Here's how the part is built. I have some questions about the finished solid (model axes, mm). A direction names the side the tool comes from. Round coordinates to 2 decimals unless told otherwise and drop trailing zeros. Write each loop counter-clockwise with the first axis right and the second up, starting at its lowest first coordinate (ties: lowest second). Pieces come first, ordered by that corner, then holes. Notation, with made-up numbers: (-35, -32.75) -> (-16, -32.75) arc R8 ccw to (-16, -23.75) -> close; hole circle Ø4 at (46.25, 55.25). An arc over 180 degrees is marked (long way). Put each result on its own line as item: value. Start each with the question number.
1. Suppose I cut it at C-C (y = -6). Please give me the cut outline in (x, z), then the cut area to 3 significant figures.
2. Suppose I cut it at B-B (y = -0.25). Please give me the cut outline in (x, z), then the cut area to 3 significant figures.
3. Which directions (+Z, -Z, +X, -X, +Y, -Y) give clear straight access to the entire face, cutting with the end or side of a thin tool? Please do faces 1 (the face through (5.51, -0.16, 2.13)), 2 (the face through (-4, -5, 7.12)), 3 (the face through (-3.99, -6.91, 8.03)), 4 (the face through (-2, 3.95, 5)), 5 (the face through (6, -3, 5)).
4. For pin 1 (0.5 mm diameter, centred on x = -1, y = 0, fed in from -Z); pin 2 (5 mm diameter, centred on x = -1, z = 3.5, fed in from -Y); pin 3 (0.8 mm diameter, centred on y = -5, z = 2.5, fed in from -X); pin 4 (1.9 mm diameter, centred on y = 1.5, z = 3.5, fed in from +X), each with a flat end and sliding along its axis, tell me the tip position at first contact or that it passes through.
5. I need wall thicknesses on probe 1 along Y at (x, z) = (1, 3); probe 2 along Y at (x, z) = (0.5, 7.5); probe 3 along Z at (x, y) = (3.5, -2.5). Which ranges of each line are inside material? Lowest first, please. Write a range as from..to.
6. We'd pull the mould along Z, two halves only. Please class faces 6 (the face through (-4, -5, 8.12)), 7 (the face through (2, 3.45, 5)), 8 (the face through (-4.5, -5.2, 7.6)): +Z half, -Z half, draft (parallel to the pull), parting line (faces both ways), or undercut.
7. Suppose I cut it at D-D (x = -4). Please give me the cut outline in (y, z), then the cut area to 3 significant figures.
8. Suppose I cut it at A-A (x = -2.75). Please give me the cut outline in (y, z).
```python
from build123d import *

# Parameters (mm, degrees)
SKIZZE3_W                       = 12
SKIZZE3_H                       = 7.9
AUFSATZ_LINEAR_AUSTRAGEN2_DEPTH = 10.16
AUFSATZ_LINEAR_AUSTRAGEN3_DEPTH = 10.16
SCHNITT_LINEAR_AUSTRAGEN1_DEPTH = 9
SKIZZE6_W                       = 1
SKIZZE6_H                       = 1
AUFSATZ_LINEAR_AUSTRAGEN4_DEPTH = 3.45
SKIZZE7_W                       = 1
SKIZZE7_H                       = 1
AUFSATZ_LINEAR_AUSTRAGEN5_DEPTH = 9
FASE1_SIZE                      = 1
FASE1_SIZE2                     = 0.176326981
FASE1_PART_2_SIZE               = 1
FASE1_PART_2_SIZE2              = 0.176326981
FASE1_PART_3_SIZE               = 1
FASE1_PART_3_SIZE2              = 0.176326981
FASE1_PART_4_SIZE               = 1
FASE1_PART_4_SIZE2              = 0.176326981
FASE1_PART_5_SIZE               = 1
FASE1_PART_5_SIZE2              = 0.176326981
FASE1_PART_6_SIZE               = 1
FASE1_PART_6_SIZE2              = 0.176326981
FASE1_PART_7_SIZE               = 1
FASE1_PART_7_SIZE2              = 0.176326981
FASE1_PART_8_SIZE               = 1
FASE1_PART_8_SIZE2              = 0.176326981
FASE14_SIZE                     = 1
FASE14_SIZE2                    = 0.176326981
FASE14_PART_2_SIZE              = 1
FASE14_PART_2_SIZE2             = 0.176326981
FASE14_PART_3_SIZE              = 1
FASE14_PART_3_SIZE2             = 0.176326981
FASE14_PART_4_SIZE              = 1
FASE14_PART_4_SIZE2             = 0.176326981
FASE14_PART_5_SIZE              = 1
FASE14_PART_5_SIZE2             = 0.176326981
FASE14_PART_6_SIZE              = 1
FASE14_PART_6_SIZE2             = 0.176326981
FASE14_PART_7_SIZE              = 1
FASE14_PART_7_SIZE2             = 0.176326981
FASE14_PART_8_SIZE              = 1
FASE14_PART_8_SIZE2             = 0.176326981
FASE15_SIZE                     = 0.1
FASE16_SIZE                     = 0.5


with BuildPart() as part:
    # Skizze3 → Aufsatz-Linear austragen2 (new body)
    with BuildSketch(Plane.XY):
        Rectangle(SKIZZE3_W, SKIZZE3_H)
    extrude(amount=AUFSATZ_LINEAR_AUSTRAGEN2_DEPTH)

    # Skizze4 → Aufsatz-Linear austragen3 (add, through all)
    with BuildSketch(Plane.XY.offset(10.16)):
        Polygon((3, 3.95), (3, 4.45), (4, 4.45), (6, 3.95), align=None)
    extrude(amount=-AUFSATZ_LINEAR_AUSTRAGEN3_DEPTH)

    # Skizze5 → Schnitt-Linear austragen1 (cut)
    with BuildSketch(Plane(origin=(6, 0, 0), x_dir=(0, 0, -1), z_dir=(1, 0, 0))):
        with BuildLine():
            Line((-9.86, 3.45), (-9.86, -1.39))
            ThreePointArc((-9.86, -1.39), (-7.602375704, -2.785098012), (-5.08, -1.96))
            ThreePointArc((-5.08, -1.96), (-2.557624296, -2.785098012), (-0.3, -1.39))
            Line((-0.3, -1.39), (-0.3, 3.45))
            Line((-0.3, 3.45), (-9.86, 3.45))
        make_face()
    extrude(amount=-SCHNITT_LINEAR_AUSTRAGEN1_DEPTH, mode=Mode.SUBTRACT)

    # Skizze6 → Aufsatz-Linear austragen4 (add)
    with BuildSketch(Plane(origin=(0, -3.95, 0), x_dir=(-1, 0, 0), z_dir=(0, -1, 0))):
        with Locations((4, -7.62)):
            Rectangle(SKIZZE6_W, SKIZZE6_H)
        with Locations((4, -2.54)):
            Rectangle(SKIZZE6_W, SKIZZE6_H)
    extrude(amount=AUFSATZ_LINEAR_AUSTRAGEN4_DEPTH)

    # Skizze7 → Aufsatz-Linear austragen5 (add)
    with BuildSketch(Plane(origin=(-3, 0, 0), x_dir=(0, 0, -1), z_dir=(1, 0, 0))):
        with Locations((-7.62, -0.15)):
            Rectangle(SKIZZE7_W, SKIZZE7_H)
        with Locations((-2.54, -0.15)):
            Rectangle(SKIZZE7_W, SKIZZE7_H)
    extrude(amount=AUFSATZ_LINEAR_AUSTRAGEN5_DEPTH)

    # Fase1
    fase1_edges = [part.edges().sort_by_distance(p)[0] for p in [
        (-3.5, -7.4, 7.62),
    ]]
    fase1_side = [part.faces().sort_by_distance(p)[0] for p in [
        (-3.5, -5.675, 7.62),
    ]]
    chamfer(fase1_edges, length=FASE1_SIZE, length2=FASE1_SIZE2, reference=fase1_side[0])

    # Fase1 part 2
    fase1_part_2_edges = [part.edges().sort_by_distance(p)[0] for p in [
        (-4, -7.4, 8.12),
    ]]
    fase1_part_2_side = [part.faces().sort_by_distance(p)[0] for p in [
        (-4, -5.675, 8.12),
    ]]
    chamfer(fase1_part_2_edges, length=FASE1_PART_2_SIZE, length2=FASE1_PART_2_SIZE2, reference=fase1_part_2_side[0])

    # Fase1 part 3
    fase1_part_3_edges = [part.edges().sort_by_distance(p)[0] for p in [
        (-4.5, -7.4, 7.62),
    ]]
    fase1_part_3_side = [part.faces().sort_by_distance(p)[0] for p in [
        (-4.5, -5.675, 7.62),
    ]]
    chamfer(fase1_part_3_edges, length=FASE1_PART_3_SIZE, length2=FASE1_PART_3_SIZE2, reference=fase1_part_3_side[0])

    # Fase1 part 4
    fase1_part_4_edges = [part.edges().sort_by_distance(p)[0] for p in [
        (-4, -7.4, 7.12),
    ]]
    fase1_part_4_side = [part.faces().sort_by_distance(p)[0] for p in [
        (-4, -5.675, 7.12),
    ]]
    chamfer(fase1_part_4_edges, length=FASE1_PART_4_SIZE, length2=FASE1_PART_4_SIZE2, reference=fase1_part_4_side[0])

    # Fase1 part 5
    fase1_part_5_edges = [part.edges().sort_by_distance(p)[0] for p in [
        (-4.5, -7.4, 2.54),
    ]]
    fase1_part_5_side = [part.faces().sort_by_distance(p)[0] for p in [
        (-4.5, -5.675, 2.54),
    ]]
    chamfer(fase1_part_5_edges, length=FASE1_PART_5_SIZE, length2=FASE1_PART_5_SIZE2, reference=fase1_part_5_side[0])

    # Fase1 part 6
    fase1_part_6_edges = [part.edges().sort_by_distance(p)[0] for p in [
        (-4, -7.4, 2.04),
    ]]
    fase1_part_6_side = [part.faces().sort_by_distance(p)[0] for p in [
        (-4, -5.675, 2.04),
    ]]
    chamfer(fase1_part_6_edges, length=FASE1_PART_6_SIZE, length2=FASE1_PART_6_SIZE2, reference=fase1_part_6_side[0])

    # Fase1 part 7
    fase1_part_7_edges = [part.edges().sort_by_distance(p)[0] for p in [
        (-3.5, -7.4, 2.54),
    ]]
    fase1_part_7_side = [part.faces().sort_by_distance(p)[0] for p in [
        (-3.5, -5.675, 2.54),
    ]]
    chamfer(fase1_part_7_edges, length=FASE1_PART_7_SIZE, length2=FASE1_PART_7_SIZE2, reference=fase1_part_7_side[0])

    # Fase1 part 8
    fase1_part_8_edges = [part.edges().sort_by_distance(p)[0] for p in [
        (-4, -7.4, 3.04),
    ]]
    fase1_part_8_side = [part.faces().sort_by_distance(p)[0] for p in [
        (-4, -5.675, 3.04),
    ]]
    chamfer(fase1_part_8_edges, length=FASE1_PART_8_SIZE, length2=FASE1_PART_8_SIZE2, reference=fase1_part_8_side[0])

    # Fase14
    fase14_edges = [part.edges().sort_by_distance(p)[0] for p in [
        (6, -0.65, 7.62),
    ]]
    fase14_side = [part.faces().sort_by_distance(p)[0] for p in [
        (1.5, -0.65, 7.62),
    ]]
    chamfer(fase14_edges, length=FASE14_SIZE, length2=FASE14_SIZE2, reference=fase14_side[0])

    # Fase14 part 2
    fase14_part_2_edges = [part.edges().sort_by_distance(p)[0] for p in [
        (6, -0.15, 8.12),
    ]]
    fase14_part_2_side = [part.faces().sort_by_distance(p)[0] for p in [
        (1.5, -0.15, 8.12),
    ]]
    chamfer(fase14_part_2_edges, length=FASE14_PART_2_SIZE, length2=FASE14_PART_2_SIZE2, reference=fase14_part_2_side[0])

    # Fase14 part 3
    fase14_part_3_edges = [part.edges().sort_by_distance(p)[0] for p in [
        (6, 0.35, 7.62),
    ]]
    fase14_part_3_side = [part.faces().sort_by_distance(p)[0] for p in [
        (1.5, 0.35, 7.62),
    ]]
    chamfer(fase14_part_3_edges, length=FASE14_PART_3_SIZE, length2=FASE14_PART_3_SIZE2, reference=fase14_part_3_side[0])

    # Fase14 part 4
    fase14_part_4_edges = [part.edges().sort_by_distance(p)[0] for p in [
        (6, -0.15, 7.12),
    ]]
    fase14_part_4_side = [part.faces().sort_by_distance(p)[0] for p in [
        (1.5, -0.15, 7.12),
    ]]
    chamfer(fase14_part_4_edges, length=FASE14_PART_4_SIZE, length2=FASE14_PART_4_SIZE2, reference=fase14_part_4_side[0])

    # Fase14 part 5
    fase14_part_5_edges = [part.edges().sort_by_distance(p)[0] for p in [
        (6, -0.15, 3.04),
    ]]
    fase14_part_5_side = [part.faces().sort_by_distance(p)[0] for p in [
        (1.5, -0.15, 3.04),
    ]]
    chamfer(fase14_part_5_edges, length=FASE14_PART_5_SIZE, length2=FASE14_PART_5_SIZE2, reference=fase14_part_5_side[0])

    # Fase14 part 6
    fase14_part_6_edges = [part.edges().sort_by_distance(p)[0] for p in [
        (6, 0.35, 2.54),
    ]]
    fase14_part_6_side = [part.faces().sort_by_distance(p)[0] for p in [
        (1.5, 0.35, 2.54),
    ]]
    chamfer(fase14_part_6_edges, length=FASE14_PART_6_SIZE, length2=FASE14_PART_6_SIZE2, reference=fase14_part_6_side[0])

    # Fase14 part 7
    fase14_part_7_edges = [part.edges().sort_by_distance(p)[0] for p in [
        (6, -0.15, 2.04),
    ]]
    fase14_part_7_side = [part.faces().sort_by_distance(p)[0] for p in [
        (1.5, -0.15, 2.04),
    ]]
    chamfer(fase14_part_7_edges, length=FASE14_PART_7_SIZE, length2=FASE14_PART_7_SIZE2, reference=fase14_part_7_side[0])

    # Fase14 part 8
    fase14_part_8_edges = [part.edges().sort_by_distance(p)[0] for p in [
        (6, -0.65, 2.54),
    ]]
    fase14_part_8_side = [part.faces().sort_by_distance(p)[0] for p in [
        (1.5, -0.65, 2.54),
    ]]
    chamfer(fase14_part_8_edges, length=FASE14_PART_8_SIZE, length2=FASE14_PART_8_SIZE2, reference=fase14_part_8_side[0])

    # Fase15
    fase15_edges = [part.edges().sort_by_distance(p)[0] for p in [
        (6, 3.45, 5.08),
        (6, -2.785098012, 7.602375704),
        (6, -2.785098012, 2.557624296),
    ]]
    chamfer(fase15_edges, length=FASE15_SIZE)

    # Fase16
    fase16_edges = [part.edges().sort_by_distance(p)[0] for p in [
        (6, -3.95, 5.08),
    ]]
    chamfer(fase16_edges, length=FASE16_SIZE)


solid = part.part
```
Verdict:
1. outline: (-4.5, 2.04) -> (-3.5, 2.04) -> (-3.5, 3.04) -> (-4.5, 3.04) -> close; (-4.5, 7.12) -> (-3.5, 7.12) -> (-3.5, 8.12) -> (-4.5, 8.12) -> close
1. area: 2.00 mm^2
2. outline: (-6, 0) -> (6, 0) -> (6, 0.3) -> (-3, 0.3) -> (-3, 2.04) -> (5, 2.04) -> (6, 2.22) -> (6, 2.86) -> (5, 3.04) -> (-3, 3.04) -> (-3, 7.12) -> (5, 7.12) -> (6, 7.3) -> (6, 7.94) -> (5, 8.12) -> (-3, 8.12) -> (-3, 9.86) -> (6, 9.86) -> (6, 10.16) -> (-6, 10.16) -> close
2. area: 53.5 mm^2
3. face 1: +X
3. face 2: +X, -X, -Y
3. face 3: +Z, +X, -X, -Y
3. face 4: +Z, -Z, -X, +Y
3. face 5: +Z, -Z, +X, +Y, -Y
4. pin 1: stops at z = 0
4. pin 2: stops at y = -3.95
4. pin 3: stops at x = -4.5
4. pin 4: stops at x = -3
5. probe 1: y = -3.95..-2.81, -0.65..0.35, 3.45..3.95
5. probe 2: y = -3.95..-2.8, -0.65..0.35, 3.45..3.95
5. probe 3: z = 0..1.57, 4.29..5.87, 8.59..10.16
6. face 6: +Z half
6. face 7: undercut
6. face 8: draft
7. outline: (-7.4, 2.22) -> (-6.4, 2.04) -> (-3.95, 2.04) -> (-3.95, 0) -> (3.95, 0) -> (3.95, 10.16) -> (-3.95, 10.16) -> (-3.95, 8.12) -> (-6.4, 8.12) -> (-7.4, 7.94) -> (-7.4, 7.3) -> (-6.4, 7.12) -> (-3.95, 7.12) -> (-3.95, 3.04) -> (-6.4, 3.04) -> (-7.4, 2.86) -> close
7. area: 86.8 mm^2
8. outline: (-3.95, 0) -> (3.95, 0) -> (3.95, 10.16) -> (-3.95, 10.16) -> close; (-0.65, 2.04) -> (0.35, 2.04) -> (0.35, 3.04) -> (-0.65, 3.04) -> close; (-0.65, 7.12) -> (0.35, 7.12) -> (0.35, 8.12) -> (-0.65, 8.12) -> close; hole (-1.96, 5.08) arc R3.15 ccw to (-1.39, 0.3) -> (3.45, 0.3) -> (3.45, 9.86) -> (-1.39, 9.86) arc R3.15 ccw to start
